```python
from build123d import *

# Parameters (mm, degrees)
F0_W     = 7
F0_H     = 7
F1_DEPTH = 6
F2_W     = 9
F2_H     = 9
F2_W_2   = 7
F2_H_2   = 7
F3_DEPTH = 1
F4_W     = 7
F4_H     = 1.5
F5_DEPTH = 1


with BuildPart() as f1:
    # F0 (on Top) → F1 (new body)
    with BuildSketch(Plane.XY):
        with Locations((-7.9846676588, 7.7618638836)):
            Rectangle(F0_W, F0_H)
    extrude(amount=F1_DEPTH)

    # F2 (on face) → F3 (join)
    with BuildSketch(Plane(origin=(0, 0, 0), x_dir=(1, 0, 0), z_dir=(0, 0, -1))):
        with Locations((-7.9846676588, -7.7618638836)):
            Rectangle(F2_W, F2_H)
        with Locations((-7.9846676588, -7.7618638836)):
            Rectangle(F2_W_2, F2_H_2, mode=Mode.SUBTRACT)
        with Locations((-7.9846676588, -7.7618638836)):
            Rectangle(F2_W_2, F2_H_2)
    extrude(amount=F3_DEPTH)

    # F4 (on face) → F5 (join)
    with BuildSketch(Plane.XY.offset(6)):
        with Locations((-7.9846676588, 5.0118638836)):
            Rectangle(F4_W, F4_H)
    extrude(amount=F5_DEPTH)


solid = f1.part
```
Read the model definition and answer for the solid it produces. Units are mm, in the model's axes. A direction names the side the tool comes from. Coordinates: 2 decimals unless noted, no trailing zeros. Loops run counter-clockwise (first coordinate to the right, second up) from the corner with the lowest first, then second, coordinate; pieces in that order, holes last.
(1) The part is cut by section D-D (y = 4). Determine the outline of the cut face in (x, z).
Solution:
outline: (-12.48, -1) - (-3.48, -1) - (-3.48, 0) - (-12.48, 0) - close
(2) The part is cut by section C-C (z = 5.25). Determine the outline of the cut face in (x, y), and give its area (3 significant figures).
Solution:
outline: (-11.48, 4.26) - (-4.48, 4.26) - (-4.48, 11.26) - (-11.48, 11.26) - close
area: 49.0 mm2
(3) A tool of negligible diameter and unlimited length cuts with its end or side. For faces 1 (the face through (-4.485, 8, 3)), 2 (the face through (-8, 9, 6)), 3 (the face through (-11.485, 8, 3)), 4 (the face through (-3.485, 7.8, -0.5)), 5 (the face through (-8, 4.262, 3)), from which of +Z, -Z, +X, -X, +Y, -Y can it reach the whole face along a straight path? Write none if from no direction.
Solution:
face 1: +Z, +X, +Y, -Y
face 2: +Z, +X, -X, +Y
face 3: +Z, -X, +Y, -Y
face 4: +Z, -Z, +X, +Y, -Y
face 5: +Z, +X, -X, -Y
(4) Consider line 1 along Z through (x, y) = (-4.25, 8); line 2 along X through (y, z) = (10, 3.5); line 3 along Z through (x, y) = (-7, 7). Determine where each line is inside the solid, lowest interval first.
Solution:
line 1: z = -1 to 0
line 2: x = -11.48 to -4.48
line 3: z = -1 to 6
(5) The part is cut by section B-B (y = 9.25). Determine the outline of the cut face in (x, z), and give its area (3 significant figures).
Solution:
outline: (-12.48, -1) - (-3.48, -1) - (-3.48, 0) - (-4.48, 0) - (-4.48, 6) - (-11.48, 6) - (-11.48, 0) - (-12.48, 0) - close
area: 51.0 mm2
(6) Flat-ended cylindrical pins translate along their axes: pin 1 Ø4 at (x, z) = (-7, 4) entering from -Y; pin 2 Ø2 at (x, z) = (-11, 1.5) entering from +Y; pin 3 Ø2.5 at (x, y) = (-9, 7.5) entering from +Z. Find the tip coordinate at first contact, or state that the pin passes through.
Solution:
pin 1: stops at y = 4.26
pin 2: stops at y = 11.26
pin 3: stops at z = 6
(7) The part is cut by section A-A (x = -5.5). Determine the outline of the cut face in (y, z), and give its area (3 significant figures).
Solution:
outline: (3.26, -1) - (12.26, -1) - (12.26, 0) - (11.26, 0) - (11.26, 6) - (5.76, 6) - (5.76, 7) - (4.26, 7) - (4.26, 0) - (3.26, 0) - close
area: 52.5 mm2
